For this review, take the finished solid that the model builds, in its own axes (mm). A direction names the side the tool comes from. Give positions to 0.01 mm unless a question says otherwise; leave off trailing zeros. Loops run counter-clockwise (first coordinate to the right, second up) from the corner with the lowest first, then second, coordinate; pieces in that order, holes last. Notation, with made-up numbers: (51.25, 19.25) - (75.25, 19.25) arc R23 cw to (75.25, 35.25) - close; hole circle Ø10 at (77.5, 62). An arc over 180 degrees is marked (long way). Use CSV: the item, a comma, the result in double quotes. Start each with the question number.
1. For faces 1 (the flat face through (7, -7, 39.878)), 2 (the cylindrical face through (-2.06, 9.3, -15.65)), list the 3-axis set-ups (+Z, -Z, +X, -X, +Y, -Y) from which the entire face can be reached by the end or side of a thin tool; tool diameter is ignored.
2. Mouldability with a two-part tool opening along X and no side actions: class faces 3 (the flat face through (7, -7, 0)), 4 (the cylindrical face through (-1.93, 8.68, 9.72)), 5 (the cylindrical face through (-3.772, -16.985, 19.66)) as pulls with the +X half, pulls with the -X half, needs draft (parallel to the pull), parting line crosses it, or undercut.
3. For pin 1 (12 mm diameter, centred on x = 13.5, y = -13, fed in from +Z); pin 2 (5 mm diameter, centred on x = -9, z = -22.5, fed in from -Y); pin 3 (3 mm diameter, centred on x = -14, z = 36, fed in from -Y), all flat-tipped, find the tip position at first contact; note any pin that passes through.
4. Take a section at C-C on z = -20. Give the boundary of the cut face in (x, y) (3 decimals).
5. Take a section at D-D on z = 25. Give the boundary of the cut face in (x, y), plus the area to 3 significant figures.
6. Take a section at A-A on y = 0. Give the boundary of the cut face in (x, z) (3 decimals), plus the area to 3 significant figures.
7. Wall thickness on line 1 (Y direction, x = 0, z = 5.5); line 2 (Y direction, x = 0, z = -12) (3 decimals): over which ranges is each line inside the solid? List them lowest first.
```python
from build123d import *

# Parameters (mm, degrees)
SKETCH1_R           = 17.399
BOSS_EXTRUDE1_DEPTH = 50.038
SKETCH3_R           = 38.1
SKETCH3_R_2         = 9.525
CUT_EXTRUDE1_DEPTH  = 10.16
SKETCH4_R           = 8.89
CUT_EXTRUDE2_DEPTH  = 127
SKETCH5_R           = 9.525
SKETCH5_R_2         = 8.89
BOSS_EXTRUDE2_DEPTH = 31.75


with BuildPart() as part:
    # Sketch1 → Boss-Extrude1 (new body)
    with BuildSketch(Plane.XY):
        Circle(SKETCH1_R)
    extrude(amount=BOSS_EXTRUDE1_DEPTH)

    # Sketch3 → Cut-Extrude1 (cut)
    with BuildSketch(Plane.XY.offset(50.038)):
        Circle(SKETCH3_R)
        Circle(SKETCH3_R_2, mode=Mode.SUBTRACT)
    extrude(amount=-CUT_EXTRUDE1_DEPTH, mode=Mode.SUBTRACT)

    # Sketch4 → Cut-Extrude2 (cut)
    with BuildSketch(Plane.XY.offset(50.038)):
        Circle(SKETCH4_R)
    extrude(amount=-CUT_EXTRUDE2_DEPTH, mode=Mode.SUBTRACT)

    # Sketch5 → Boss-Extrude2 (add)
    with BuildSketch(Plane(origin=(0, 0, 0), x_dir=(-1, 0, 0), z_dir=(0, 0, -1))):
        with Locations(Location((0, 0, 0), (0, 0, 180))):
            Circle(SKETCH5_R)
        with Locations(Location((0, 0, 0), (0, 0, 180))):
            Circle(SKETCH5_R_2, mode=Mode.SUBTRACT)
    extrude(amount=BOSS_EXTRUDE2_DEPTH)


solid = part.part
```
Check result:
1,face 1,"+Z"
1,face 2,"-Z"
2,face 3,"needs draft"
2,face 4,"undercut"
2,face 5,"parting line crosses it"
3,pin 1,"stops at z = 39.88"
3,pin 2,"stops at y = -6.96"
3,pin 3,"stops at y = -12.1"
4,outline,"circle Ø19.05 at (0, 0); hole circle Ø17.78 at (0, 0)"
5,outline,"circle Ø34.8 at (0, 0); hole circle Ø17.78 at (0, 0)"
5,area,"703 mm²"
6,outline,"(-17.399, 0) - (-9.525, 0) - (-9.525, -31.75) - (-8.89, -31.75) - (-8.89, 50.038) - (-9.525, 50.038) - (-9.525, 39.878) - (-17.399, 39.878) - close; (8.89, -31.75) - (9.525, -31.75) - (9.525, 0) - (17.399, 0) - (17.399, 39.878) - (9.525, 39.878) - (9.525, 50.038) - (8.89, 50.038) - close"
6,area,"732 mm²"
7,line 1,"y = -17.4 to -8.89, 8.89 to 17.4"
7,line 2,"y = -9.525 to -8.89, 8.89 to 9.525"
